Can you work these out from the model? Positions are in its coordinate system, mm. A direction names the side the tool comes from. Coordinates: 2 decimals unless noted, no trailing zeros. Order: outer loops, then holes, each group sorted by start corner. A loop starts at its lowest first (then second) coordinate and runs counter-clockwise, first axis right, second up.
```python
from build123d import *

# Parameters (mm, degrees)
BOSS_EXTRUDE1_DEPTH = 30
CUT_EXTRUDE2_DEPTH  = 50
CUT_EXTRUDE6_DEPTH  = 27
SHELL3_T            = 5
BOSS_EXTRUDE3_DEPTH = 20
BOSS_EXTRUDE4_START = -3
BOSS_EXTRUDE4_DEPTH = 5
SKETCH7_R           = 7.5
CUT_EXTRUDE3_DEPTH  = 2.5


with BuildPart() as part:
    # Sketch1 → Boss-Extrude1 (new body)
    with BuildSketch(Plane(origin=(0, 0, 0), x_dir=(1, 0, 0), z_dir=(0, 1, 0))):
        Polygon((-10, 60), (10, 60), (25, 10), (-25, 10), align=None)
    extrude(amount=BOSS_EXTRUDE1_DEPTH)

    # Sketch3 → Cut-Extrude2 (cut)
    with BuildSketch(Plane(origin=(-25, 0, 0), x_dir=(0, -1, 0), z_dir=(-1, 0, 0))):
        Polygon((-30, -10), (-27.26731497, -10), (-20, -60), (-30, -60), align=None)
        Polygon((0, -60), (0, -10), (-2.73268503, -10), (-10, -60), align=None)
    extrude(amount=-CUT_EXTRUDE2_DEPTH, mode=Mode.SUBTRACT)

    # Sketch10 → Cut-Extrude6 (cut)
    with BuildSketch(Plane(origin=(0, 27.26731497, 0), x_dir=(-1, 0, 0), z_dir=(0, 1, 0))):
        with BuildLine():
            Line((-22, -10), (22, -10))
            ThreePointArc((22, -10), (0, -19.112698372), (-22, -10))
        make_face()
    extrude(amount=-CUT_EXTRUDE6_DEPTH, mode=Mode.SUBTRACT)

    # Shell3 (no face opened: a closed hollow body)
    add(offset(amount=-SHELL3_T, mode=Mode.PRIVATE), mode=Mode.SUBTRACT)

    # Sketch5 → Boss-Extrude3 (add)
    with BuildSketch(Plane(origin=(-10, 0, 0), x_dir=(0, -1, 0), z_dir=(1, 0, 0))):
        with BuildLine():
            Line((-10, 60), (-8.960811725, 52.850259833))
            ThreePointArc((-8.960811725, 52.850259833), (-6.536467075, 61.023474826), (-15, 60))
            Line((-15, 60), (-10, 60))
        make_face()
    extrude(amount=BOSS_EXTRUDE3_DEPTH)

    # Sketch6 → Boss-Extrude4 (add)
    with BuildSketch(Plane(origin=(-25, 0, 0), x_dir=(0, -1, 0), z_dir=(-1, 0, 0)).offset(BOSS_EXTRUDE4_START)):
        with BuildLine():
            Line((-25.046773104, -9.993090655), (-25.046773104, -13.993090655))
            Line((-25.046773104, -13.993090655), (-5.046773104, -13.993090655))
            Line((-5.046773104, -13.993090655), (-5.046773104, -9.993090655))
            Line((-5.046773104, -9.993090655), (-5.046773104, -2.5))
            ThreePointArc((-5.046773104, -2.5), (-15.046773104, 7.5), (-25.046773104, -2.5))
            Line((-25.046773104, -2.5), (-25.046773104, -9.993090655))
        make_face()
    boss_extrude4 = extrude(amount=BOSS_EXTRUDE4_DEPTH)

    # Sketch7 → Cut-Extrude3 (cut)
    with BuildSketch(Plane(origin=(-22, 0, 0), x_dir=(0, 0, -1), z_dir=(1, 0, 0))):
        with Locations((1.25, 15.046773104)):
            Circle(SKETCH7_R)
    cut_extrude3 = extrude(amount=-CUT_EXTRUDE3_DEPTH, mode=Mode.SUBTRACT)

    # Mirror2: Boss-Extrude4, Cut-Extrude3 across plane
    add(boss_extrude4.mirror(Plane.ZY))
    add(cut_extrude3.mirror(Plane.ZY), mode=Mode.SUBTRACT)


solid = part.part
```
1. Imagine slicing it at A-A on x = -3. Please give me the cut outline in (y, z).
Completed:
outline: (4.04, -18.97) - (8.96, -52.85) arc R5.1 ccw (long way) to (15, -60) - (20, -60) - (25.96, -18.97) - close; hole (9.82, -23.99) - (14.33, -55) - (15.67, -55) - (20.18, -23.99) - close
2. Imagine slicing it at D-D on z = -51.5. Please give me the cut outline in (x, y), then the cut area to 3 significant figures.
Completed:
outline: (-12.55, 8.76) - (12.55, 8.76) - (12.55, 21.24) - (-12.55, 21.24) - close; hole (-7.33, 13.82) - (7.33, 13.82) - (7.33, 16.18) - (-7.33, 16.18) - close
area: 278 mm2
3. Please list where these lines run through material, in increasing order: probe 1 along X at (y, z) = (14.5, 1.5); probe 2 along X at (y, z) = (10.5, -10); probe 3 along Y at (x, z) = (-23.8, -1.25).
Completed:
probe 1: x = -27 to -24.5, 24.5 to 27
probe 2: x = -27 to -22, 22 to 27
probe 3: y = 5.13 to 7.55, 22.55 to 24.97
4. Imagine slicing it at B-B on y = 17.5. Please give me the cut outline in (x, z).
Completed:
outline: (-27, -13.99) - (-23.8, -13.99) - (-10, -60) - (10, -60) - (23.8, -13.99) - (27, -13.99) - (27, 7.19) - (22, 7.19) - (22, 5.84) - (24.5, 5.84) - (24.5, -8.34) - (22, -8.34) - (22, -10) arc R31.11 cw to (-22, -10) - (-22, -8.34) - (-24.5, -8.34) - (-24.5, 5.84) - (-22, 5.84) - (-22, 7.19) - (-27, 7.19) - close; hole (-16.79, -19.97) - (-10.05, -42.44) - (10.05, -42.44) - (16.79, -19.97) arc R36.11 cw to start
5. On a 3-axis mill with a long thin cutter (end or side, diameter ignored), from which of +Z, -Z, +X, -X, +Y, -Y can I reach the whole of each face in a straight line? I mean faces 5 (the flat face through (24, 4, -10)), 6 (the flat face through (25, 15, -13.993)), 7 (the cylindrical face through (23.232, 7.725, 0.376)), 8 (the flat face through (10, 9, -59)). Say none if no direction works.
Completed:
face 5: +Z, +X, -X, -Y
face 6: -Z, +X, +Y, -Y
face 7: none
face 8: -Z, +X, -Y
6. I'm going to push flat-ended pins straight in: pin 1 (3 mm diameter, centred on x = 8.5, y = 6, fed in from -Z); pin 2 (2.5 mm diameter, centred on x = 24, y = 26.5, fed in from +Z); pin 3 (8 mm diameter, centred on x = -14, z = -36.5, fed in from -Y); pin 4 (5.5 mm diameter, centred on x = 24, z = -10.5, fed in from +Y). Where does each tip first touch, or does it pass through?
Completed:
pin 1: stops at z = -61.91
pin 2: stops at z = -10
pin 3: stops at y = 6
pin 4: stops at y = 27.27
7. Thinking about a two-plate mould opening in Y: for faces 1 (the flat face through (22, 15, -9)), 2 (the flat face through (-0.235, 11.745, -37.241)), 3 (the cylindrical face through (-0.24, 15.08, -24.11)), 4 (the cylindrical face through (24.465, 14.827, 7.498)), which applies, pulls with the +Y half, pulls with the -Y half, needs draft (parallel to the pull), parting line crosses it, or undercut?
Completed:
face 1: needs draft
face 2: undercut
face 3: undercut
face 4: parting line crosses it
8. Imagine slicing it at C-C on z = -1.25. Please give me the cut outline in (x, y).
Completed:
outline: (-27, 5.13) - (-22, 5.13) - (-22, 7.55) - (-24.5, 7.55) - (-24.5, 22.55) - (-22, 22.55) - (-22, 24.97) - (-27, 24.97) - close; (22, 5.13) - (27, 5.13) - (27, 24.97) - (22, 24.97) - (22, 22.55) - (24.5, 22.55) - (24.5, 7.55) - (22, 7.55) - close
